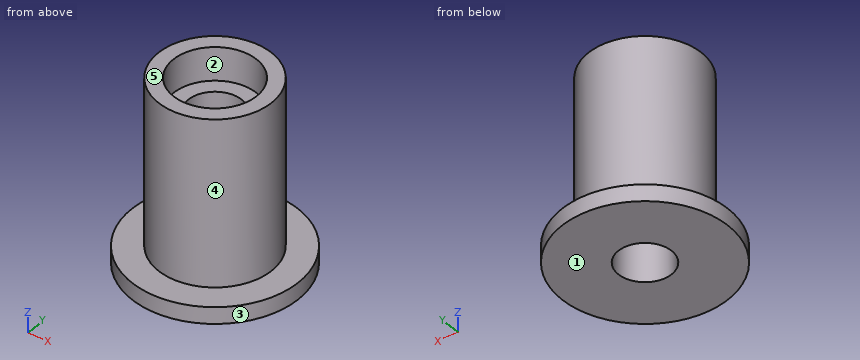
from build123d import *

# Parameters (mm, degrees)
SKETCH1_R           = 5
SKETCH1_R_2         = 1.6
BOSS_EXTRUDE1_DEPTH = 1
SKETCH1_3_R         = 3.4
SKETCH1_3_R_2       = 2.5
BOSS_EXTRUDE2_DEPTH = 10
SKETCH1_4_R         = 2.5
SKETCH1_4_R_2       = 1.6
BOSS_EXTRUDE3_DEPTH = 8


with BuildPart() as part:
    # Sketch1 → Boss-Extrude1 (new body)
    with BuildSketch(Plane.XY):
        Circle(SKETCH1_R)
        Circle(SKETCH1_R_2, mode=Mode.SUBTRACT)
    extrude(amount=-BOSS_EXTRUDE1_DEPTH)

    # Sketch1<3> → Boss-Extrude2 (add)
    with BuildSketch(Plane.XY):
        Circle(SKETCH1_3_R)
        Circle(SKETCH1_3_R_2, mode=Mode.SUBTRACT)
    extrude(amount=BOSS_EXTRUDE2_DEPTH)

    # Sketch1<4> → Boss-Extrude3 (add)
    with BuildSketch(Plane.XY):
        Circle(SKETCH1_4_R)
        Circle(SKETCH1_4_R_2, mode=Mode.SUBTRACT)
    extrude(amount=BOSS_EXTRUDE3_DEPTH)


solid = part.part
The listing builds one solid part. Answer for the finished solid, in the listing's coordinates (mm). Face numbers are marked on the shaded views. A direction names the side the tool comes from. Round coordinates to 2 decimals unless told otherwise and drop trailing zeros. Order: outer loops, then holes, each group sorted by start corner. A loop starts at its lowest first (then second) coordinate and runs counter-clockwise, first axis right, second up. Notation, with made-up numbers: (-7, 36) -> (6, 36) arc R20 ccw to (6, 53) -> close; hole circle Ø4 at (61, -20.75). An arc over 180 degrees is marked (long way). One line per item, written item: value.
Item 1: Straight lines are drawn through the part: L1, parallel to Y at x = 0, z = 9.15; L2, parallel to Y at x = 0, z = 6; L3, parallel to Z at x = -2.25, y = 3.5. For each, find the intervals that lie inside material, in ascending order.
Taken from the geometry:
L1: y = -3.4 to -2.5, 2.5 to 3.4
L2: y = -3.4 to -1.6, 1.6 to 3.4
L3: z = -1 to 0
Item 2: Find section A-A, the plane y = 0. Give the vertices of the cut face in (x, z).
Taken from the geometry:
outline: (-5, -1) -> (-1.6, -1) -> (-1.6, 8) -> (-2.5, 8) -> (-2.5, 10) -> (-3.4, 10) -> (-3.4, 0) -> (-5, 0) -> close; (1.6, -1) -> (5, -1) -> (5, 0) -> (3.4, 0) -> (3.4, 10) -> (2.5, 10) -> (2.5, 8) -> (1.6, 8) -> close
Item 3: For the marked faces 4 and 5, determine the directions among +Z, -Z, +X, -X, +Y, -Y from which every point of the face is accessible in a straight line to the end or side of a thin tool.
Taken from the geometry:
face 4: +Z
face 5: +Z, +X, -X, +Y, -Y
Item 4: Given P1, Ø6, axis at x = -2, z = 4, coming from the -Y side; P2, Ø3, axis at x = -3.5, z = 2, coming from the -Y side; P3, Ø1.5, axis at x = -1, y = -1, coming from the +Z side; P4, Ø2.5, axis at x = 0, y = 0, coming from the -Z side, each flat-ended and moving along its own axis, determine where each tip first touches the part or whether it passes through.
Taken from the geometry:
P1: stops at y = -3.4
P2: stops at y = -2.75
P3: stops at z = 8
P4: passes through
Item 5: For a pull along X with two mould halves and no side action, classify the marked faces 1, 2 and 3 as released by +X, released by -X, zero draft, split by the parting line, or undercut.
Taken from the geometry:
face 1: zero draft
face 2: undercut
face 3: split by the parting line
Item 6: Find section C-C, the plane z = 8.5. Give the vertices of the cut face in (x, y).
Taken from the geometry:
outline: circle Ø6.8 at (0, 0); hole circle Ø5 at (0, 0)
Item 7: Find section D-D, the plane y = -3. Give the vertices of the cut face in (x, z), then the cut area to 3 significant figures.
Taken from the geometry:
outline: (-4, -1) -> (4, -1) -> (4, 0) -> (1.6, 0) -> (1.6, 10) -> (-1.6, 10) -> (-1.6, 0) -> (-4, 0) -> close
area: 40.0 mm2
